```python
from build123d import *

# Parameters (mm, degrees)
SKETCH2_W           = 65
SKETCH2_H           = 50
EXTRUDE_5_DEPTH     = 42
SKETCH3_W           = 110
SKETCH3_H           = 31
CUT_EXTRUDE1_DEPTH  = 50
SKETCH4_R           = 2.5
CUT_EXTRUDE2_DEPTH  = 50
SKETCH5_W           = 65
SKETCH5_H           = 15
CUT_EXTRUDE3_DEPTH  = 50
SKETCH6_W           = 65
SKETCH6_H           = 4.5
CUT_EXTRUDE4_DEPTH  = 50
SKETCH7_W           = 65
SKETCH7_H           = 35
BOSS_EXTRUDE2_DEPTH = 5
FILLET1_R           = 5
FILLET2_R           = 6
SKETCH8_W           = 65
SKETCH8_H           = 15
BOSS_EXTRUDE3_DEPTH = 5
FILLET3_R           = 3
SKETCH9_R           = 2.5
CUT_EXTRUDE5_DEPTH  = 5
CUT_EXTRUDE6_DEPTH  = 5
SKETCH11_W          = 5
SKETCH11_H          = 86.5
CUT_EXTRUDE8_DEPTH  = 71


with BuildPart() as part:
    # Sketch2 → Extrude 5 (new body)
    with BuildSketch(Plane(origin=(0, 0, 0), x_dir=(1, 0, 0), z_dir=(0, 1, 0))):
        Rectangle(SKETCH2_W, SKETCH2_H)
    extrude(amount=EXTRUDE_5_DEPTH)

    # Sketch3 → Cut-Extrude1 (cut)
    with BuildSketch(Plane.XY.offset(25)):
        with Locations((-32.5, 21)):
            Rectangle(SKETCH3_W, SKETCH3_H)
    extrude(amount=-CUT_EXTRUDE1_DEPTH, mode=Mode.SUBTRACT)

    # Sketch4 → Cut-Extrude2 (cut)
    with BuildSketch(Plane(origin=(0, 42, 0), x_dir=(1, 0, 0), z_dir=(0, 1, 0))):
        with Locations((-17.5, 0)):
            Circle(SKETCH4_R)
    extrude(amount=-CUT_EXTRUDE2_DEPTH, mode=Mode.SUBTRACT)

    # Sketch5 → Cut-Extrude3 (cut)
    with BuildSketch(Plane(origin=(0, 42, 0), x_dir=(1, 0, 0), z_dir=(0, 1, 0))):
        with Locations((0, -17.5)):
            Rectangle(SKETCH5_W, SKETCH5_H)
    extrude(amount=-CUT_EXTRUDE3_DEPTH, mode=Mode.SUBTRACT)

    # Sketch6 → Cut-Extrude4 (cut)
    with BuildSketch(Plane(origin=(0, 42, 0), x_dir=(1, 0, 0), z_dir=(0, 1, 0))):
        with Locations((0, 22.75)):
            Rectangle(SKETCH6_W, SKETCH6_H)
    extrude(amount=-CUT_EXTRUDE4_DEPTH, mode=Mode.SUBTRACT)

    # Sketch7 → Boss-Extrude2 (add)
    with BuildSketch(Plane(origin=(0, 0, -20.5), x_dir=(-1, 0, 0), z_dir=(0, 0, -1))):
        with Locations((0, -12)):
            Rectangle(SKETCH7_W, SKETCH7_H)
    extrude(amount=-BOSS_EXTRUDE2_DEPTH)

    # Fillet1
    fillet1_edges = [part.edges().sort_by_distance(p)[0] for p in [
        (22.5, 5.5, -5.25),
        (22.5, 36.5, -5.25),
    ]]
    fillet(fillet1_edges, radius=FILLET1_R)

    # Fillet2
    fillet2_edges = [part.edges().sort_by_distance(p)[0] for p in [
        (0, 0, -15.5),
    ]]
    fillet(fillet2_edges, radius=FILLET2_R)

    # Sketch8 → Boss-Extrude3 (add)
    with BuildSketch(Plane(origin=(0, 0, -20.5), x_dir=(-1, 0, 0), z_dir=(0, 0, -1))):
        with Locations((0, 49.5)):
            Rectangle(SKETCH8_W, SKETCH8_H)
    extrude(amount=-BOSS_EXTRUDE3_DEPTH)

    # Fillet3
    fillet3_edges = [part.edges().sort_by_distance(p)[0] for p in [
        (0, 42, -15.5),
    ]]
    fillet(fillet3_edges, radius=FILLET3_R)

    # Sketch9 → Cut-Extrude5 (cut)
    with BuildSketch(Plane.XY.offset(-15.5)):
        with Locations((-22.5, 49.5)):
            Circle(SKETCH9_R)
        with Locations((-0.5, 49.5)):
            Circle(SKETCH9_R)
        with Locations((21.5, 49.5)):
            Circle(SKETCH9_R)
    extrude(amount=-CUT_EXTRUDE5_DEPTH, mode=Mode.SUBTRACT)

    # Sketch10 → Cut-Extrude6 (cut)
    with BuildSketch(Plane.XY.offset(-15.5)):
        with BuildLine():
            Line((-24.75, -23.440008753), (-24.75, -20.559991247))
            ThreePointArc((-24.75, -20.559991247), (-22.5, -18.309991247), (-20.25, -20.559991247))
            Line((-20.25, -20.559991247), (-20.25, -23.440008753))
            ThreePointArc((-20.25, -23.440008753), (-22.5, -25.690008753), (-24.75, -23.440008753))
        make_face()
        with BuildLine():
            Line((-2.75, -23.440008753), (-2.75, -20.559991247))
            ThreePointArc((-2.75, -20.559991247), (-0.5, -18.309991247), (1.75, -20.559991247))
            Line((1.75, -20.559991247), (1.75, -23.440008753))
            ThreePointArc((1.75, -23.440008753), (-0.5, -25.690008753), (-2.75, -23.440008753))
        make_face()
        with BuildLine():
            Line((19.25, -23.440008753), (19.25, -20.559991247))
            ThreePointArc((19.25, -20.559991247), (21.5, -18.309991247), (23.75, -20.559991247))
            Line((23.75, -20.559991247), (23.75, -23.440008753))
            ThreePointArc((23.75, -23.440008753), (21.5, -25.690008753), (19.25, -23.440008753))
        make_face()
    extrude(amount=-CUT_EXTRUDE6_DEPTH, mode=Mode.SUBTRACT)

    # Sketch11 → Cut-Extrude8 (cut)
    with BuildSketch(Plane.XY.offset(10)):
        with Locations((30, 13.75)):
            Rectangle(SKETCH11_W, SKETCH11_H)
    extrude(amount=-CUT_EXTRUDE8_DEPTH, mode=Mode.SUBTRACT)


solid = part.part
```
For this review, take the finished solid that the model builds, in its own axes (mm). A direction names the side the tool comes from. Round coordinates to 2 decimals unless told otherwise and drop trailing zeros. Write each loop counter-clockwise with the first axis right and the second up, starting at its lowest first coordinate (ties: lowest second). Pieces come first, ordered by that corner, then holes. Notation, with made-up numbers: (58, 72) - (98, 72) arc R17 ccw to (98, 85) - close; hole circle Ø4 at (16, 27.5). An arc over 180 degrees is marked (long way). Answer as CSV lines item,"result". Start each with the question number.
(1) Add section D-D, the plane x = -28. State the section outline as (y, z) points, plus the area to 3 significant figures.
(2) For pin 1 (6 mm diameter, centred on x = -17.5, z = 0, fed in from +Y); pin 2 (6.5 mm diameter, centred on y = 23.5, z = -3, fed in from -X); pin 3 (6 mm diameter, centred on x = 21.5, y = 49.5, fed in from +Z); pin 4 (12 mm diameter, centred on y = -19.5, z = -11.5, fed in from -X), all flat-tipped, find the tip position at first contact; note any pin that passes through.
(3) Mouldability with a two-part tool opening along Y and no side actions: class faces 1 (the flat face through (27.5, 23, -5)), 2 (the flat face through (-2, 57, -18)), 3 (the flat face through (23.75, -22, -18)) as +Y half, -Y half, draft (parallel to the pull), parting line (faces both ways), or undercut.
(4) Add section A-A, the plane x = 21.5. State the section outline as (y, z) points, plus the area to 3 significant figures.
(5) Add section C-C, the plane z = 0. State the section outline as (x, y) points, plus the area to 3 significant figures.
(6) Add section B-B, the plane y = 49.5. State the section outline as (x, z) points.
(7) For line 1 (X direction, y = 38, z = 0); line 2 (Y direction, x = 21.5, z = -18.8); line 3 (Y direction, x = 0.5, z = 7.5), list the stretches that pass through material, from the lowest coordinate up.
(8) Machinability: for faces 4 (the cylindrical face through (21, 35.07, -5.46)), 5 (the flat face through (-3, 0, 0)), 6 (the flat face through (-2, 52, -15.5)), 7 (the cylindrical face through (21.45, -18.31, -17.96)), 8 (the cylindrical face through (-20, 39, 0)), which of the approach directions +Z, -Z, +X, -X, +Y, -Y give a long, thin tool a straight path to every point of the face, cutting with its end or side? Answer none if there is none.
From the geometry:
1,outline,"(-29.5, -20.5) - (5.5, -20.5) - (5.5, 10) - (0, 10) - (0, -9.5) arc R6 cw to (-6, -15.5) - (-29.5, -15.5) - close; (36.5, -20.5) - (57, -20.5) - (57, -15.5) - (45, -15.5) arc R3 cw to (42, -12.5) - (42, 10) - (36.5, 10) - close"
1,area,"568 mm²"
2,pin 1,"stops at y = 42"
2,pin 2,"stops at x = 22.5"
2,pin 3,"stops at z = -15.5"
2,pin 4,"stops at x = -32.5"
3,face 1,"draft"
3,face 2,"+Y half"
3,face 3,"undercut"
4,outline,"(-29.5, -20.5) - (-25.69, -20.5) - (-25.69, -15.5) - (-29.5, -15.5) - close; (-18.31, -20.5) - (7.5, -20.5) - (7.5, 10) - (0, 10) - (0, -9.5) arc R6 cw to (-6, -15.5) - (-18.31, -15.5) - close; (34.5, -20.5) - (47, -20.5) - (47, -15.5) - (45, -15.5) arc R3 cw to (42, -12.5) - (42, 10) - (34.5, 10) - close; (52, -20.5) - (57, -20.5) - (57, -15.5) - (52, -15.5) - close"
4,area,"628 mm²"
5,outline,"(-32.5, 0) - (-20, 0) - (-20, 5.5) - (-32.5, 5.5) - close; (-32.5, 36.5) - (-20, 36.5) - (-20, 42) - (-32.5, 42) - close; (-15, 0) - (27.5, 0) - (27.5, 42) - (-15, 42) - (-15, 36.5) - (17.5, 36.5) arc R5 cw to (22.5, 31.5) - (22.5, 10.5) arc R5 cw to (17.5, 5.5) - (-15, 5.5) - close"
5,area,"771 mm²"
6,outline,"(-32.5, -20.5) - (-25, -20.5) - (-25, -15.5) - (-32.5, -15.5) - close; (-20, -20.5) - (-3, -20.5) - (-3, -15.5) - (-20, -15.5) - close; (2, -20.5) - (19, -20.5) - (19, -15.5) - (2, -15.5) - close; (24, -20.5) - (27.5, -20.5) - (27.5, -15.5) - (24, -15.5) - close"
7,line 1,"x = -32.5 to -20, -15 to 27.5"
7,line 2,"y = -29.5 to -25.69, -18.31 to 7.5, 34.5 to 47, 52 to 57"
7,line 3,"y = 0 to 5.5, 36.5 to 42"
8,face 4,"+Z, -Z, -X"
8,face 5,"+Z, +X, -X, -Y"
8,face 6,"+Z, +X, -X, +Y"
8,face 7,"+Z, -Z"
8,face 8,"+Y, -Y"
